Build history of the part. All positions in model axes, mm. A direction names the side the tool comes from. Round coordinates to 2 decimals unless told otherwise and drop trailing zeros. Write each loop counter-clockwise with the first axis right and the second up, starting at its lowest first coordinate (ties: lowest second). Pieces come first, ordered by that corner, then holes.
Item 1: Mould opens along Y. For faces 4 (the flat face through (30.283, 7, -2)), 5 (the flat face through (27, 2.372, -3)), 6 (the flat face through (31.683, 7, -2)), 7 (the flat face through (28, 3.772, -2)) say: +Y half, -Y half, draft (parallel to the pull), parting line (faces both ways), or undercut.
Item 2: Wall check: probe 1 along Y at (x, z) = (28, 0.05); probe 2 along X at (y, z) = (6.75, -2.5); probe 3 along Y at (x, z) = (30, -3.3). Give the ranges that are in metal, low to high.
Item 3: Band-saw the part on D-D, the plane z = -2.25. Write the cut outline in (x, y).
Item 4: Band-saw the part on A-A, the plane y = 5.25. Write the cut outline in (x, z), then the cut area to 3 significant figures.
Item 5: Band-saw the part on C-C, the plane z = -0.05. Write the cut outline in (x, y).
Item 6: 3-axis set-ups, long thin cutter, end or side, ignore diameter. For faces 1 (the flat face through (21.683, 7, -2)), 2 (the flat face through (27, 10.972, -2)), 3 (the cylindrical face through (27.446, 3.062, -1.483)): which of +Z, -Z, +X, -X, +Y, -Y reach the whole face in a straight line?
Item 7: Band-saw the part on B-B, the plane x = 29. Write the cut outline in (y, z), then the cut area to 3 significant figures.
Autodesk Inventor part; units mm, degrees
ref_plane "作業平面2" through (3.1146, -16.3784, -3.723) normal (0, 0, 1) x (1, 0, 0)
ref_plane "YZ Plane" through (0, 0, 0) normal (1, 0, 0) x (0, 1, 0)
ref_plane "XZ Plane" through (0, 0, 0) normal (0, 1, 0) x (-1, 0, 0)
ref_plane "作業平面1" through (26.683, 7.3716, 0.277) normal (0, 0, 1) x (0, -1, 0)
ref_plane "作業平面2" through (3.1146, -16.3784, -3.723) normal (0, 0, 1) x (1, 0, 0)
sketch "スケッチ1" plane through (26.683, 7.3716, 0.277) normal (0, 0, 1) x (0, -1, 0)
  arc A0 (0.9652, -1.8217) -> (0.7443, -1.8564) centre (0.9303, -2.3204) ccw
  arc A1 (0.7443, 1.8564) -> (0.7443, -1.8564) centre (0, 0) ccw
  arc A2 (0.7443, 1.8564) -> (0.9652, 1.8217) centre (0.9303, 2.3204) ccw
  arc A3 (1.5, 1.3229) -> (0.9652, 1.8217) centre (1, 1.3229) ccw
  line L0 (1.5, 1.3229) -> (1.5, -1.3229)
  arc A4 (0.9652, -1.8217) -> (1.5, -1.3229) centre (1, -1.3229) ccw
  arc A5 (2, -3.5) -> (3.5, -2) centre (2, -2) ccw
  line L1 (3.5, -2) -> (3.5, 2)
  arc A6 (3.5, 2) -> (2, 3.5) centre (2, 2) ccw
  line L2 (2, 3.5) -> (-2, 3.5)
  arc A7 (-2, 3.5) -> (-3.5, 2) centre (-2, 2) ccw
  line L3 (-3.5, 2) -> (-3.5, -2)
  arc A8 (-3.5, -2) -> (-2, -3.5) centre (-2, -2) ccw
  line L4 (-2, -3.5) -> (2, -3.5)
  line L5 (5, -5) -> (-5, -5)
  line L6 (-5, -5) -> (-5, 5)
  line L7 (-5, 5) -> (5, 5)
  line L8 (5, 5) -> (5, -5)
  line L9 (5, -5) -> (-5, 5) construction
  line L10 (-5, -5) -> (5, 5) construction
  line L11 (3.6, -3.6) -> (-3.6, -3.6)
  line L12 (-3.6, -3.6) -> (-3.6, 3.6)
  line L13 (-3.6, 3.6) -> (3.6, 3.6)
  line L14 (3.6, 3.6) -> (3.6, -3.6)
  line L15 (3.6, -3.6) -> (-3.6, 3.6) construction
  line L16 (-3.6, -3.6) -> (3.6, 3.6) construction
  point P0 (7.3716, -26.683)
  dimension "d0" = 0.1
  dimension "d1" = 10
extrude "押し出し1" add sketch "スケッチ1" against normal up to surface (4 mm away) contours L5 L6 L7 L8
fillet "フィレット1" radius 2 4 edges at (31.683, 12.3716, -1.723) (21.683, 12.3716, -1.723) (21.683, 2.3716, -1.723) (31.683, 2.3716, -1.723)
sketch "スケッチ3" plane through (23.683, 2.3716, 0.277) normal (0, -1, 0) x (1, 0, 0)
  line L0 (6, 0) -> (6, -4)
  line L1 (0, 0) -> (6, 0)
  line L2 (0, -4) -> (0, 0)
  circle A0 centre (3, -2) radius 0.8
  line L3 (6, -4) -> (0, -4)
  line L4 (0, 0) -> (6, -4) construction
  line L5 (0, -4) -> (6, 0) construction
  point P0 (-23.683, -0.277)
  point P1 (6, -3.5)
  point P2 (3, -2)
  dimension "d11" = 1.6
extrude "押し出し3" cut sketch "スケッチ3" against normal blind 4 contours A0
properties part number "Tap_zigu"
Results:
1. face 4: undercut
1. face 5: -Y half
1. face 6: draft
1. face 7: undercut
2. probe 1: y = 2.37 to 3.77, 10.97 to 12.37
2. probe 2: x = 21.68 to 23.08, 30.28 to 31.68
2. probe 3: y = 2.4 to 3.77, 10.97 to 12.35
3. outline: (21.68, 4.37) arc R2 ccw to (23.68, 2.37) - (26.08, 2.37) - (26.08, 3.77) - (23.08, 3.77) - (23.08, 10.97) - (30.28, 10.97) - (30.28, 3.77) - (27.28, 3.77) - (27.28, 2.37) - (29.68, 2.37) arc R2 ccw to (31.68, 4.37) - (31.68, 10.37) arc R2 ccw to (29.68, 12.37) - (23.68, 12.37) arc R2 ccw to (21.68, 10.37) - close
4. outline: (21.68, -3.72) - (23.08, -3.72) - (23.08, 0.28) - (21.68, 0.28) - close; (30.28, -3.72) - (31.68, -3.72) - (31.68, 0.28) - (30.28, 0.28) - close
4. area: 11.2 mm2
5. outline: (21.68, 4.37) arc R2 ccw to (23.68, 2.37) - (29.68, 2.37) arc R2 ccw to (31.68, 4.37) - (31.68, 10.37) arc R2 ccw to (29.68, 12.37) - (23.68, 12.37) arc R2 ccw to (21.68, 10.37) - close; hole (23.08, 3.77) - (30.28, 3.77) - (30.28, 10.97) - (23.08, 10.97) - close
6. face 1: +Z, -Z, -X, +Y, -Y
6. face 2: +Z, -Z
6. face 3: -Y
7. outline: (2.37, -3.72) - (3.77, -3.72) - (3.77, 0.28) - (2.37, 0.28) - close; (10.97, -3.72) - (12.37, -3.72) - (12.37, 0.28) - (10.97, 0.28) - close
7. area: 11.2 mm2
